CAD build for the part. Positions are in the model's coordinates, mm. A direction names the side the tool comes from. Coordinates: 2 decimals unless noted, no trailing zeros. Order: outer loops, then holes, each group sorted by start corner. A loop starts at its lowest first (then second) coordinate and runs counter-clockwise, first axis right, second up. Notation, with made-up numbers: M 9,-34 L 52,-34 A5 cw 52,-30 Z; hole C 71.25,89.5 d4. An arc over 180 degrees is marked long. One line per item, written item: value.
from build123d import *

# Parameters (mm, degrees)
F0_R     = 14.2875
F1_DEPTH = 25.4
F2_DEPTH = 25.4
F3_DEPTH = 55.118


with BuildPart() as f1:
    # F0 (on Front) → F1 (new body)
    with BuildSketch(Plane.XZ):
        with BuildLine():
            Line((9.5121844836, 26.9452959039), (0, 28.575))
            ThreePointArc((0, 28.575), (-28.575, 0), (0, -28.575))
            Line((0, -28.575), (9.5121844836, -26.9452959039))
            ThreePointArc((9.5121844836, -26.9452959039), (23.3274655355, -16.5033322905), (28.575, 0))
            ThreePointArc((28.575, 0), (23.3274655355, 16.5033322905), (9.5121844836, 26.9452959039))
        make_face()
        with BuildLine():
            ThreePointArc((-13.4703841816, 4.7625), (0, 14.2875), (13.4703841816, 4.7625))
            Line((13.4703841816, 4.7625), (19.05, 4.7625))
            Line((19.05, 4.7625), (19.05, -4.7625))
            Line((19.05, -4.7625), (13.4703841816, -4.7625))
            ThreePointArc((13.4703841816, -4.7625), (0, -14.2875), (-13.4703841816, -4.7625))
            Line((-13.4703841816, -4.7625), (-19.05, -4.7625))
            Line((-19.05, -4.7625), (-19.05, 4.7625))
            Line((-19.05, 4.7625), (-13.4703841816, 4.7625))
        make_face(mode=Mode.SUBTRACT)
        with BuildLine():
            Line((57.1919272622, 18.7764181619), (9.5121844836, 26.9452959039))
            ThreePointArc((9.5121844836, 26.9452959039), (23.3274655355, 16.5033322905), (28.575, 0))
            ThreePointArc((28.575, 0), (23.3274655355, -16.5033322905), (9.5121844836, -26.9452959039))
            Line((9.5121844836, -26.9452959039), (57.1919272622, -18.7764181619))
            ThreePointArc((57.1919272622, -18.7764181619), (34.925, 0), (57.1919272622, 18.7764181619))
        make_face()
        with BuildLine():
            ThreePointArc((73.025, 0), (68.5383952831, 12.2804730295), (57.1919272622, 18.7764181619))
            ThreePointArc((57.1919272622, 18.7764181619), (34.925, 0), (57.1919272622, -18.7764181619))
            ThreePointArc((57.1919272622, -18.7764181619), (68.5383952831, -12.2804730295), (73.025, 0))
        make_face()
        with Locations((53.975, 0)):
            Circle(F0_R, mode=Mode.SUBTRACT)
    extrude(amount=F1_DEPTH)

    # F0 (on Front) → F2 (join)
    with BuildSketch(Plane.XZ):
        with BuildLine():
            ThreePointArc((-13.4703841816, -4.7625), (-14.2875, 0), (-13.4703841816, 4.7625))
            Line((-13.4703841816, 4.7625), (-19.05, 4.7625))
            Line((-19.05, 4.7625), (-19.05, -4.7625))
            Line((-19.05, -4.7625), (-13.4703841816, -4.7625))
        make_face()
    extrude(amount=F2_DEPTH)

    # F0 (on Front) → F3 (join)
    with BuildSketch(Plane.XZ):
        with BuildLine():
            Line((9.5121844836, 26.9452959039), (0, 28.575))
            ThreePointArc((0, 28.575), (-28.575, 0), (0, -28.575))
            Line((0, -28.575), (9.5121844836, -26.9452959039))
            ThreePointArc((9.5121844836, -26.9452959039), (23.3274655355, -16.5033322905), (28.575, 0))
            ThreePointArc((28.575, 0), (23.3274655355, 16.5033322905), (9.5121844836, 26.9452959039))
        make_face()
        with BuildLine():
            ThreePointArc((-13.4703841816, 4.7625), (0, 14.2875), (13.4703841816, 4.7625))
            Line((13.4703841816, 4.7625), (19.05, 4.7625))
            Line((19.05, 4.7625), (19.05, -4.7625))
            Line((19.05, -4.7625), (13.4703841816, -4.7625))
            ThreePointArc((13.4703841816, -4.7625), (0, -14.2875), (-13.4703841816, -4.7625))
            Line((-13.4703841816, -4.7625), (-19.05, -4.7625))
            Line((-19.05, -4.7625), (-19.05, 4.7625))
            Line((-19.05, 4.7625), (-13.4703841816, 4.7625))
        make_face(mode=Mode.SUBTRACT)
        with BuildLine():
            ThreePointArc((-13.4703841816, -4.7625), (-14.2875, 0), (-13.4703841816, 4.7625))
            Line((-13.4703841816, 4.7625), (-19.05, 4.7625))
            Line((-19.05, 4.7625), (-19.05, -4.7625))
            Line((-19.05, -4.7625), (-13.4703841816, -4.7625))
        make_face()
    extrude(amount=F3_DEPTH)


solid = f1.part
Q1. Which spindle directions (+Z, -Z, +X, -X, +Y, -Y) get a long thin tool onto all of the face, cutting with end or side? Do faces 1 (the face through (16, -27, 4.762)), 2 (the face through (-13, -55.118, 7)). Say none if no direction does.
Recorded:
face 1: +Y, -Y
face 2: +Z, -Z, +X, -X, -Y
Q2. Slice it at B-B (x = 58.5). List the corners of the cut face in (y, z).
Recorded:
outline: M -25.4,-18.5 L 0,-18.5 L 0,-13.55 L -25.4,-13.55 Z; M -25.4,13.55 L 0,13.55 L 0,18.5 L -25.4,18.5 Z
Q3. Pin check, flat tips, straight feed: pin 1 Ø1.7 at (x, y) = (17, -35.5) entering from +Z; pin 2 Ø6 at (x, y) = (15.5, -16) entering from -Z; pin 3 Ø2 at (y, z) = (-26, -8.5) entering from +X; pin 4 Ø8 at (x, y) = (-1, -32.5) entering from +Z (3 decimals). Stop position of each tip, or through.
Recorded:
pin 1: stops at z = 23.57
pin 2: stops at z = -26.43
pin 3: stops at x = 71.4
pin 4: stops at z = 28.575
Q4. Slice it at D-D (y = -22). Give the number of separate pieces and of enclosed holes in the cut face, plus the area to 3 significant figures.
Recorded:
separate pieces: 1
enclosed holes: 2
area: 3,110 mm^2
Q5. Slice it at C-C (z = 6.5). List the corners of the cut face in (x, y).
Recorded:
outline: M -27.83,-55.12 L -12.72,-55.12 L -12.72,0 L -27.83,0 Z; M 12.72,-55.12 L 27.83,-55.12 L 27.83,-25.4 L 41.25,-25.4 L 41.25,0 L 12.72,0 Z; M 66.7,-25.4 L 71.88,-25.4 L 71.88,0 L 66.7,0 Z
Q6. Drill centre lines: line 1 along Y through (x, z) = (40.5, 19.5); line 2 along X through (y, z) = (-4.5, 1); line 3 along X through (y, z) = (-27, 9.5). Where is each one in solid material? Low to high.
Recorded:
line 1: y = -25.4 to 0
line 2: x = -28.56 to -14.25, 19.05 to 39.72, 68.23 to 73
line 3: x = -26.95 to -10.67, 10.67 to 26.95
Q7. Mould opens along Z. For faces 3 (the face through (-28.57, -27.17, 0.63)), 4 (the face through (67.6, -12.5, 4.3)), 5 (the face through (22, 0, 0)) say: released by +Z, released by -Z, zero draft, split by the parting line, or undercut.
Recorded:
face 3: split by the parting line
face 4: undercut
face 5: zero draft
